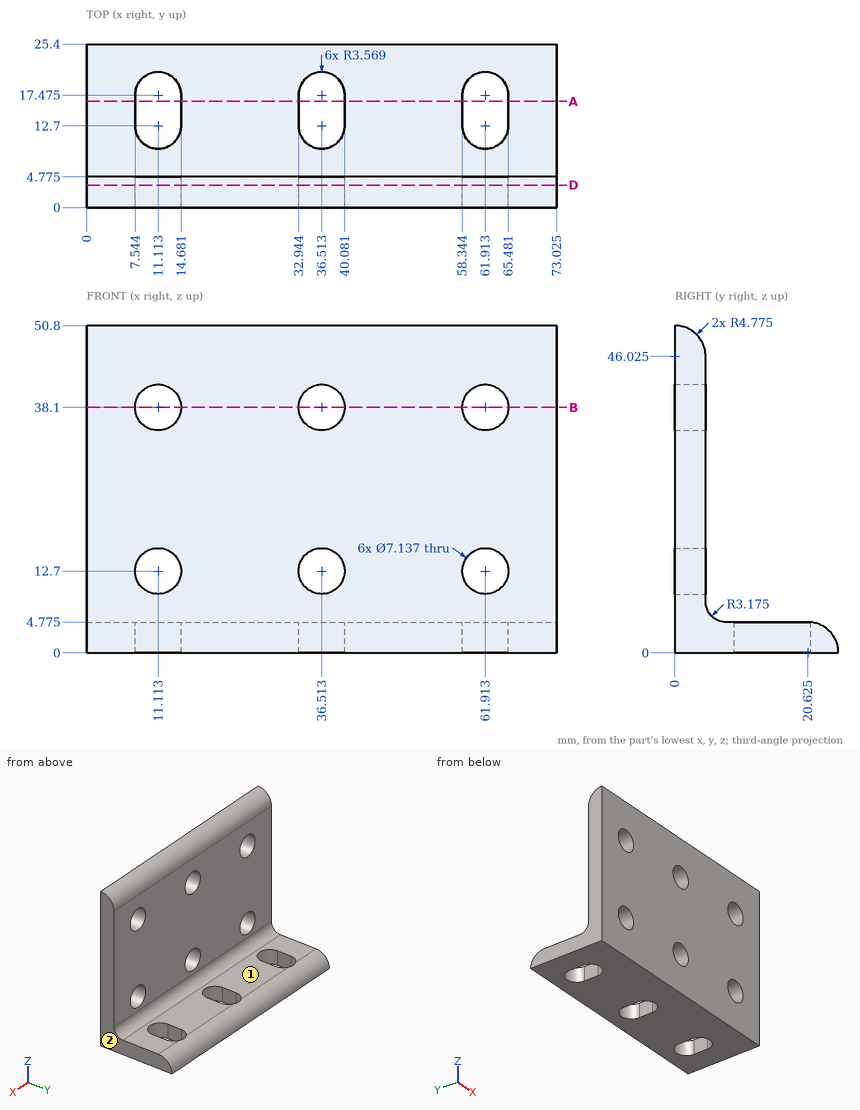
Answer from the drawing. Dimensions are ordinates in mm from the lowest x, y and z of the part. A direction names the side the tool comes from. Round coordinates to 2 decimals unless told otherwise and drop trailing zeros. Order: outer loops, then holes, each group sorted by start corner. A loop starts at its lowest first (then second) coordinate and runs counter-clockwise, first axis right, second up. Notation, with made-up numbers: (-24.75, 17.25) - (6.25, 17.25) arc R11 ccw to (6.25, 26.25) - close; hole circle Ø3 at (75.25, 80.25). An arc over 180 degrees is marked (long way). Put each result on its own line as item: value. Start each with the question number.
(1) For the marked faces 1 and 2, determine the directions among +Z, -Z, +X, -X, +Y, -Y from which every point of the face is accessible in a straight line to the end or side of a thin tool.
(2) Straight lines are drawn through the part: probe 1 along X at (y, z) = (1.8, 38.1) (1 decimal); probe 2 along Z at (x, y) = (44, 9.5) (1 decimal). For each, find the intervals that lie inside material, in ascending order. Write a range as from..to.
(3) Given P1, Ø8, axis at x = 36.51, z = 12.7, coming from the +Y side (1 decimal); P2, Ø2, axis at x = 58, y = 6.5, coming from the +Z side; P3, Ø1.5, axis at x = 14.5, y = 17.5, coming from the +Z side (1 decimal); P4, Ø1.5, axis at x = 25, z = 34.5, coming from the -Y side, each flat-ended and moving along its own axis, determine where each tip first touches the part or whether it passes through.
(4) Find section A-A (y = 16.5). Give the vertices of the cut face in (x, z) (1 decimal).
(5) Find section D-D (y = 3.5). Give the vertices of the cut face in (x, z) (1 decimal), plus the area to 3 significant figures.
Reply:
1. face 1: +Z, +X, -X, +Y
1. face 2: +Z, -Z, +X, +Y, -Y
2. probe 1: 0..7.5, 14.7..32.9, 40.1..58.3, 65.5..73
2. probe 2: 0..4.8
3. P1: y = 4.8
3. P2: z = 5.93
3. P3: z = 4.8
3. P4: y = 0
4. outline: (0, 0) - (7.5, 0) - (7.5, 4.8) - (0, 4.8) - close; (14.7, 0) - (32.9, 0) - (32.9, 4.8) - (14.7, 4.8) - close; (40.1, 0) - (58.3, 0) - (58.3, 4.8) - (40.1, 4.8) - close; (65.5, 0) - (73, 0) - (73, 4.8) - (65.5, 4.8) - close
5. outline: (0, 0) - (73, 0) - (73, 49.3) - (0, 49.3) - close; hole circle Ø7.1 at (11.1, 12.7); hole circle Ø7.1 at (11.1, 38.1); hole circle Ø7.1 at (36.5, 12.7); hole circle Ø7.1 at (36.5, 38.1); hole circle Ø7.1 at (61.9, 12.7); hole circle Ø7.1 at (61.9, 38.1)
5. area: 3,360 mm^2
